The drawing under review shows one solid part. Ordinate dimensions are in mm from its lowest x, y, z. Coordinates: 2 decimals unless noted, no trailing zeros. Loops run counter-clockwise (first coordinate to the right, second up) from the corner with the lowest first, then second, coordinate; pieces in that order, holes last.
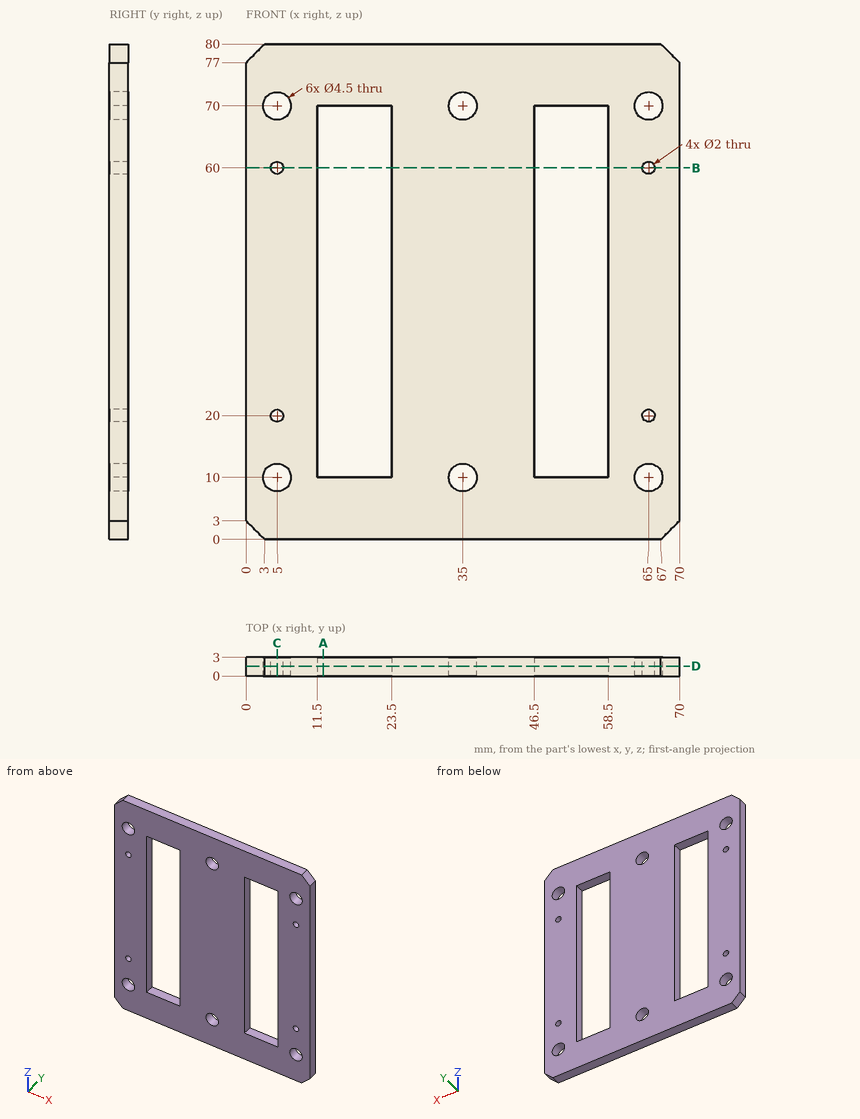
Q1. For line 1 (X direction, y = 2.3, z = 20); line 2 (X direction, y = 1.05, z = 65.5); line 3 (Z direction, x = 16, y = 1.1), list the stretches that pass through material, from the lowest coordinate up.
Q2. Take a section at D-D, the plane y = 1.6. Give the number of separate pieces and of enclosed holes in the cut face, then the cut area to 3 significant figures.
Q3. Take a section at B-B, the plane z = 60. Write out the cut boundary in (x, y).
Q4. Take a section at C-C, the plane x = 5. Write out the cut boundary in (y, z).
Q5. Take a section at A-A, the plane x = 12.5. Write out the cut boundary in (y, z).
Entries:
1. line 1: x = 0 to 4, 6 to 11.5, 23.5 to 46.5, 58.5 to 64, 66 to 70
1. line 2: x = 0 to 11.5, 23.5 to 46.5, 58.5 to 70
1. line 3: z = 0 to 10, 70 to 80
2. separate pieces: 1
2. enclosed holes: 12
2. area: 4,030 mm2
3. outline: (0, 0) - (4, 0) - (4, 3) - (0, 3) - close; (6, 0) - (11.5, 0) - (11.5, 3) - (6, 3) - close; (23.5, 0) - (46.5, 0) - (46.5, 3) - (23.5, 3) - close; (58.5, 0) - (64, 0) - (64, 3) - (58.5, 3) - close; (66, 0) - (70, 0) - (70, 3) - (66, 3) - close
4. outline: (0, 0) - (3, 0) - (3, 7.75) - (0, 7.75) - close; (0, 12.25) - (3, 12.25) - (3, 19) - (0, 19) - close; (0, 21) - (3, 21) - (3, 59) - (0, 59) - close; (0, 61) - (3, 61) - (3, 67.75) - (0, 67.75) - close; (0, 72.25) - (3, 72.25) - (3, 80) - (0, 80) - close
5. outline: (0, 0) - (3, 0) - (3, 10) - (0, 10) - close; (0, 70) - (3, 70) - (3, 80) - (0, 80) - close
